The listing builds one solid part. Answer for the finished solid, in the listing's coordinates (mm). Face numbers are marked on the shaded views. Coordinates: 2 decimals unless noted, no trailing zeros. Order: outer loops, then holes, each group sorted by start corner. A loop starts at its lowest first (then second) coordinate and runs counter-clockwise, first axis right, second up. Notation, with made-up numbers: M 41,-5 L 57,-5 A21 ccw 57,7 Z; hole C -12.75,80.25 d9. An arc over 180 degrees is marked long. One line per item, written item: value. Start each with the question number.
Q1. The part is cut by section C-C on y = -193.5. Give the vertices of the cut face in (x, z), then the cut area to 4 significant figures.
Q2. The part is cut by section B-B on y = -290. Give the vertices of the cut face in (x, z), then the cut area to 4 significant figures.
Q3. Straight lines are drawn through the part: line 1 along X through (y, z) = (-132, 18.5); line 2 along Z through (x, y) = (-50.7, -290); line 3 along Z through (x, y) = (-58, -103). For each, find the intervals that lie inside material, in ascending order. Write a range as [from, to].
Q4. The part is cut by section A-A on z = 11.25. Give the vertices of the cut face in (x, y), then the cut area to 3 significant figures.
Q5. Determine the mould class of the marked faces 1, 2 and 3 for opening direction Z: pulls with the +Z half, pulls with the -Z half, needs draft (parallel to the pull), parting line crosses it, or undercut.
Q6. The part is cut by section D-D on x = -69.5. Give the vertices of the cut face in (y, z).
Q7. This flat-tipped pin is pushed along its axis until it touches: pin 1 Ø10 at (x, y) = (-64, -97) entering from +Z. Where does it stop, or does it pass through?
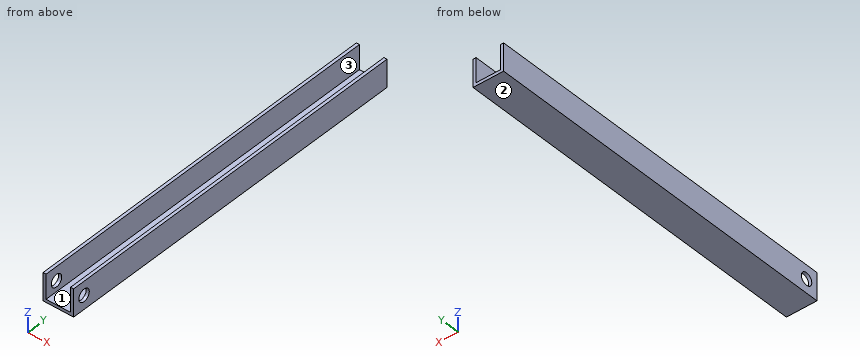
```python
from build123d import *

# Parameters (mm, degrees)
F1_DEPTH = 300
F4_R     = 5
F5_DEPTH = 84


with BuildPart() as f1:
    # F0 (on Front) → F1 (new body)
    with BuildSketch(Plane.XZ):
        Polygon((-74.9858543277, 22.5), (-74.9858543277, 0), (-49.9858543277, 0), (-49.9858543277, 22.5), (-52.4858543277, 22.5), (-52.4858543277, 20), (-52.4858543277, 2.5), (-72.4858543277, 2.5), (-72.4858543277, 20), (-72.4858543277, 22.5), align=None)
    extrude(amount=F1_DEPTH)

    # F4 (on offset) → F5 (cut)
    with BuildSketch(Plane.YZ.offset(-24.9858543277)):
        with Locations((-290, 11.25)):
            Circle(F4_R)
    extrude(amount=-F5_DEPTH, mode=Mode.SUBTRACT)


solid = f1.part
```
Output:
1. outline: M -74.99,0 L -49.99,0 L -49.99,22.5 L -52.49,22.5 L -52.49,2.5 L -72.49,2.5 L -72.49,22.5 L -74.99,22.5 Z
1. area: 162.5 mm^2
2. outline: M -74.99,0 L -49.99,0 L -49.99,6.25 L -52.49,6.25 L -52.49,2.5 L -72.49,2.5 L -72.49,6.25 L -74.99,6.25 Z; M -74.99,16.25 L -72.49,16.25 L -72.49,22.5 L -74.99,22.5 Z; M -52.49,16.25 L -49.99,16.25 L -49.99,22.5 L -52.49,22.5 Z
2. area: 112.5 mm^2
3. line 1: x = [-74.99, -72.49], [-52.49, -49.99]
3. line 2: z = [0, 6.25], [16.25, 22.5]
3. line 3: z = [0, 2.5]
4. outline: M -74.99,-300 L -72.49,-300 L -72.49,-295 L -74.99,-295 Z; M -74.99,-285 L -72.49,-285 L -72.49,0 L -74.99,0 Z; M -52.49,-300 L -49.99,-300 L -49.99,-295 L -52.49,-295 Z; M -52.49,-285 L -49.99,-285 L -49.99,0 L -52.49,0 Z
4. area: 1,450 mm^2
5. face 1: pulls with the +Z half
5. face 2: pulls with the -Z half
5. face 3: needs draft
6. outline: M -300,0 L 0,0 L 0,2.5 L -300,2.5 Z
7. pin 1: stops at z = 2.5
